Source: CAD feature listing. Evaluate the final solid. Frame: model axes, mm. Face numbers are marked on the shaded views. A direction names the side the tool comes from. Coordinates: 2 decimals unless noted, no trailing zeros. Order: outer loops, then holes, each group sorted by start corner. A loop starts at its lowest first (then second) coordinate and runs counter-clockwise, first axis right, second up.
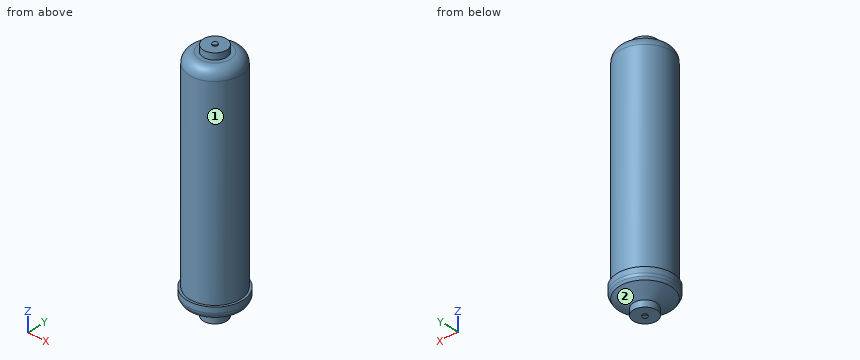
```python
from build123d import *

# Parameters (mm, degrees)
FILLET1_R = 12.7
FILLET2_R = 6.35


with BuildPart() as part:
    # Sketch1 → Revolve1 (revolve)
    with BuildSketch(Plane(origin=(0, 0, 0), x_dir=(0, 0, -1), z_dir=(1, 0, 0))):
        Polygon((0, 0), (0, 3.175), (-1.27, 3.175), (-1.27, 14.732), (-9.398, 14.732), (-20.32, 32.555084127), (-24.892, 35.306), (-33.7566, 35.306), (-33.7566, 32.512), (-299.4152, 32.512), (-299.4152, 14.732), (-307.594, 14.732), (-307.594, 3.175), (-308.864, 3.175), (-308.864, 0), align=None)
    revolve(axis=Axis((0, 0, 0), (0, 0, 1)))

    # Fillet1
    fillet1_edges = [part.edges().sort_by_distance(p)[0] for p in [
        (0, -32.512, 299.4152),
    ]]
    fillet(fillet1_edges, radius=FILLET1_R)

    # Fillet2
    fillet2_edges = [part.edges().sort_by_distance(p)[0] for p in [
        (0, -35.306, 24.892),
    ]]
    fillet(fillet2_edges, radius=FILLET2_R)


solid = part.part
```
Q1. Set-up query: the marked faces 1 and 2. Return all of +Z, -Z, +X, -X, +Y, -Y with unobstructed straight access to the full face (end or side cutting, diameter ignored); none if empty.
Solutions:
face 1: +Z
face 2: -Z
Q2. Material intervals for line 1 along Z through (x, y) = (-8, 11); line 2 along X through (y, z) = (-1.5, 177); line 3 along Y through (x, z) = (-28.5, 111), sorted ascending.
Solutions:
line 1: z = 1.27 to 307.59
line 2: x = -32.48 to 32.48
line 3: y = -15.65 to 15.65
Q3. Pin query (flat end, axial travel): P1, Ø6, axis at x = -24.5, z = 121, coming from the +Y side; P2, Ø1, axis at y = -25.5, z = 102, coming from the +X side; P3, Ø3, axis at x = 16, z = 47.5, coming from the +Y side. Return the tip coordinate at first contact, or that it passes through.
Solutions:
P1: stops at y = 24.39
P2: stops at x = 20.79
P3: stops at y = 29.1
Q4. Section query A-A on z = 68.5. Output: boundary loops of the cut face in (x, y), plus the area to 3 significant figures.
Solutions:
outline: circle Ø65.02 at (0, 0)
area: 3,320 mm2
